```python
from build123d import *

# Parameters (mm, degrees)
F1_DEPTH = 19.05
F2_R     = 3.81
F3_DEPTH = 25.4
F4_R     = 3.81
F5_DEPTH = 25.4


with BuildPart() as f1:
    # F0 (on Top) → F1 (new body)
    with BuildSketch(Plane.XY):
        with BuildLine():
            Line((-3.175, 19.555938), (-3.175, 41.152703))
            ThreePointArc((-3.175, 41.152703), (-6.369333, 40.780599), (-9.525, 40.160926))
            Line((-9.525, 40.160926), (-9.525, 28.730926))
            Line((-9.525, 28.730926), (-29.633756, 28.730926))
            ThreePointArc((-29.633756, 28.730926), (-30.714503, 27.572539), (-31.75, 26.373531))
            Line((-31.75, 26.373531), (-31.75, -26.373531))
            ThreePointArc((-31.75, -26.373531), (0, -41.275), (31.75, -26.373531))
            Line((31.75, -26.373531), (31.75, 26.373531))
            ThreePointArc((31.75, 26.373531), (30.714503, 27.572539), (29.633756, 28.730926))
            Line((29.633756, 28.730926), (9.525, 28.730926))
            Line((9.525, 28.730926), (9.525, 40.160926))
            ThreePointArc((9.525, 40.160926), (6.369333, 40.780599), (3.175, 41.152703))
            Line((3.175, 41.152703), (3.175, 19.555938))
            ThreePointArc((3.175, 19.555938), (0, -19.812), (-3.175, 19.555938))
        make_face()
    extrude(amount=F1_DEPTH)

    # F2 (on face) → F3 (cut)
    with BuildSketch(Plane.XY.offset(19.05)):
        with Locations((25.4, 0)):
            Circle(F2_R)
        with Locations((-25.4, 0)):
            Circle(F2_R)
    extrude(amount=-F3_DEPTH, mode=Mode.SUBTRACT)

    # F4 (on face) → F5 (cut)
    with BuildSketch(Plane.YZ.offset(9.525)):
        with Locations((34.802703, 9.525)):
            Circle(F4_R)
    extrude(amount=-F5_DEPTH, mode=Mode.SUBTRACT)


solid = f1.part
```
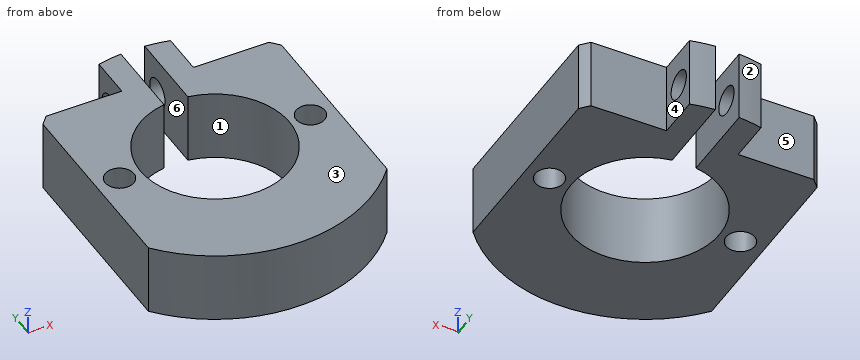
Geometry: final body of the model. Coordinates: model frame, mm. Face numbers are marked on the shaded views. A direction names the side the tool comes from. Coordinates: 2 decimals unless noted, no trailing zeros. Write each loop counter-clockwise with the first axis right and the second up, starting at its lowest first coordinate (ties: lowest second). Pieces come first, ordered by that corner, then holes. Notation, with made-up numbers: M 65.25,44.25 L 114.25,44.25 A22 ccw 114.25,64.25 Z; hole C -30.5,15.5 d6. An arc over 180 degrees is marked long. Answer as CSV lines item,"result". Start each with the question number.
Q1. Cut plane A-A on z = 7.25. Count the separate pieces of the cut face and the enclosed holes in it, then the cut area to 3 significant figures.
Q2. Pin query (flat end, axial travel): P1, Ø4, axis at x = -14, z = 9.5, coming from the -Y side; P2, Ø6, axis at x = 25.4, y = 0, coming from the -Z side; P3, Ø10, axis at y = 34.8, z = 9.52, coming from the -X side (3 decimals); P4, Ø5.5, axis at x = -22.5, z = 13.5, coming from the +Y side. Return the tip coordinate at first contact, or that it passes through.
Q3. Reachability of the marked faces 4, 5 and 6 from +Z, -Z, +X, -X, +Y, -Y: full face, straight path, thin tool, end or side. Return the list, or none.
Q4. Cut plane C-C on x = 8. Return the cut outline in (y, z) (3 decimals).
Q5. Mould query, pull axis X, two halves, no side actions, for the marked faces 1, 2 and 3. Classes: released by +X, released by -X, zero draft, split by the parting line, or undercut.
Q6. Cut plane D-D on x = 17. Return the cut outline in (y, z), then the cut area to 3 significant figures.
Q7. Line query: line 1 (X direction, y = 2.5, z = 17.5); line 2 (X direction, y = 34.5, z = 3.75) (3 decimals); line 3 (X direction, y = -15.5, z = 13.5). Output: solid intervals per line, ascending. Write a range as from..to.
Q8. Cut plane B-B on y = 0. Return the cut outline in (x, z).
Findings below:
1,separate pieces,"3"
1,enclosed holes,"2"
1,area,"2,850 mm2"
2,P1,"stops at y = -39.49"
2,P2,"passes through"
2,P3,"stops at x = -9.525"
2,P4,"stops at y = 28.73"
3,face 4,"+Z, -Z, +X, +Y"
3,face 5,"+Z, -Z, -X, +Y"
3,face 6,"+Z, -Z, +Y"
4,outline,"M -40.492,0 L -18.125,0 L -18.125,19.05 L -40.492,19.05 Z; M 18.125,0 L 40.492,0 L 40.492,19.05 L 18.125,19.05 Z; hole C 34.803,9.525 d7.62"
5,face 1,"undercut"
5,face 2,"released by -X"
5,face 3,"zero draft"
6,outline,"M -37.61,0 L -10.17,0 L -10.17,19.05 L -37.61,19.05 Z; M 10.17,0 L 28.73,0 L 28.73,19.05 L 10.17,19.05 Z"
6,area,"876 mm2"
7,line 1,"x = -31.75..-28.28, -22.52..-19.65, 19.65..22.52, 28.28..31.75"
7,line 2,"x = -9.525..-3.175, 3.175..9.525"
7,line 3,"x = -31.75..-12.34, 12.34..31.75"
8,outline,"M -31.75,0 L -29.21,0 L -29.21,19.05 L -31.75,19.05 Z; M -21.59,0 L -19.81,0 L -19.81,19.05 L -21.59,19.05 Z; M 19.81,0 L 21.59,0 L 21.59,19.05 L 19.81,19.05 Z; M 29.21,0 L 31.75,0 L 31.75,19.05 L 29.21,19.05 Z"
